Check sheet for the modelled part. Datum: model origin and axes. Units: mm. Face numbers are marked on the shaded views. Give positions to 0.01 mm unless a question says otherwise; leave off trailing zeros. Order: outer loops, then holes, each group sorted by start corner. A loop starts at its lowest first (then second) coordinate and runs counter-clockwise, first axis right, second up.
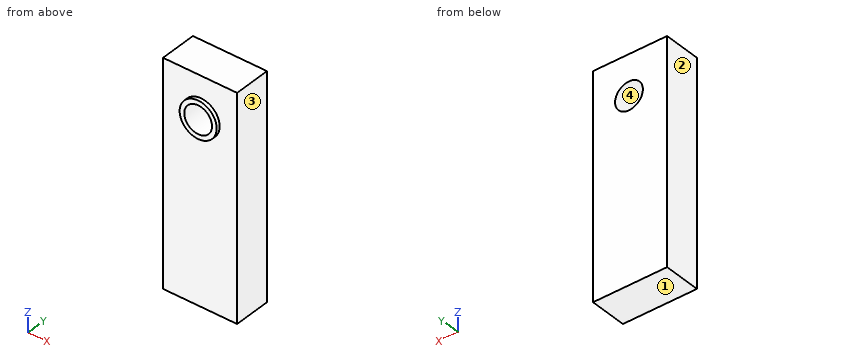
from build123d import *

# Parameters (mm, degrees)
F0_W     = 50.8
F0_H     = 25.4
F1_DEPTH = 152.4
F2_R     = 9.525
F3_DEPTH = 25.4
F4_R     = 12.7
F4_R_2   = 9.525
F5_DEPTH = 2.54


with BuildPart() as f1:
    # F0 (on Top) → F1 (new body)
    with BuildSketch(Plane.XY):
        with Locations((-25.4, -12.7)):
            Rectangle(F0_W, F0_H)
    extrude(amount=F1_DEPTH)

    # F2 (on face) → F3 (cut)
    with BuildSketch(Plane.XZ.offset(25.4)):
        with Locations((-24.664951, 124.869779)):
            Circle(F2_R)
    extrude(amount=-F3_DEPTH, mode=Mode.SUBTRACT)

    # F4 (on face) → F5 (join)
    with BuildSketch(Plane.XZ.offset(25.4)):
        with Locations((-24.664951, 124.869779)):
            Circle(F4_R)
        with Locations((-24.664951, 124.869779)):
            Circle(F4_R_2, mode=Mode.SUBTRACT)
    extrude(amount=F5_DEPTH)


solid = f1.part
1) Section check A-A, the plane x = -27. Record the cut outline in (y, z).
Recorded:
outline: (-27.94, 112.39) - (-25.4, 112.39) - (-25.4, 0) - (0, 0) - (0, 115.64) - (-27.94, 115.64) - close; (-27.94, 134.1) - (0, 134.1) - (0, 152.4) - (-25.4, 152.4) - (-25.4, 137.35) - (-27.94, 137.35) - close
2) Section check B-B, the plane z = 127. Record the cut outline in (x, y), then the cut area to 3 significant figures.
Recorded:
outline: (-50.8, -25.4) - (-37.19, -25.4) - (-37.19, -27.94) - (-33.95, -27.94) - (-33.95, 0) - (-50.8, 0) - close; (-15.38, -27.94) - (-12.14, -27.94) - (-12.14, -25.4) - (0, -25.4) - (0, 0) - (-15.38, 0) - close
area: 835 mm2
3) Section check D-D, the plane z = 96.5. Record the cut outline in (x, y), then the cut area to 3 significant figures.
Recorded:
outline: (-50.8, -25.4) - (0, -25.4) - (0, 0) - (-50.8, 0) - close
area: 1,290 mm2
4) Section check C-C, the plane y = -12.75. Record the cut outline in (x, z) (3 decimals), then the cut area to 3 significant figures.
Recorded:
outline: (-50.8, 0) - (0, 0) - (0, 152.4) - (-50.8, 152.4) - close; hole circle Ø19.05 at (-24.665, 124.87)
area: 7,460 mm2
5) Material ranges on L1, parallel to Y at x = -18, z = 98; L2, parallel to Z at x = -23.5, y = -26; L3, parallel to Z at x = -28.5, y = -6.25, recorded low to high.
Recorded:
L1: y = -25.4 to 0
L2: z = 112.22 to 115.42, 134.32 to 137.52
L3: z = 0 to 116.15, 133.59 to 152.4
6) Depth check by flat-ended pin: pin 1 Ø2 at (x, z) = (-6, 95) entering from +Y; pin 2 Ø1 at (x, z) = (-41.5, 93.5) entering from -Y. Enter the tip coordinate at first touch or a pass-through.
Recorded:
pin 1: stops at y = 0
pin 2: stops at y = -25.4
7) Draft check along X on the marked faces 1, 2, 3 and 4. Enter one of: +X half, -X half, draft (parallel to the pull), parting line (faces both ways), or undercut.
Recorded:
face 1: draft
face 2: -X half
face 3: +X half
face 4: undercut
